Autodesk Inventor part; units mm, degrees
ref_plane "YZ Plane" through (0, 0, 0) normal (1, 0, 0) x (0, 1, 0)
ref_plane "XZ Plane" through (0, 0, 0) normal (0, 1, 0) x (-1, 0, 0)
ref_plane "XY Plane" through (0, 0, 0) normal (0, 0, 1) x (1, 0, 0)
sketch "Sketch1" plane through (0, 0, 0) normal (0, 0, 1) x (1, 0, 0)
  line L0 (0, 273.8452) -> (193.6378, 193.6378) construction
  line L1 (193.6378, 193.6378) -> (273.8452, 0) construction
  line L2 (273.8452, 0) -> (193.6378, -193.6378) construction
  line L3 (193.6378, -193.6378) -> (0, -273.8452) construction
  line L4 (0, -273.8452) -> (-193.6378, -193.6378) construction
  line L5 (-193.6378, -193.6378) -> (-273.8452, 0) construction
  line L6 (-273.8452, 0) -> (-193.6378, 193.6378) construction
  line L7 (-193.6378, 193.6378) -> (0, 273.8452)
  line L8 (-193.6378, 193.6378) -> (0, 273.8452)
  line L9 (-459.9272, 770.6562) -> (-219.7185, 870.1539)
  line L10 (-96.8189, 233.7415) -> (-339.8229, 820.405) construction
  line L11 (-219.7185, 870.1539) -> (0, 870.1539)
  line L12 (0, 870.1539) -> (0, 273.8452)
  line L13 (-459.9272, 770.6562) -> (-615.2917, 615.2917)
  line L14 (-615.2917, 615.2917) -> (-193.6378, 193.6378)
  point P0 (0, 0)
  point P1 (0, 0)
  dimension "d0" = 506
  dimension "d2" = 260
  dimension "d3" = 635
extrude "Extrusion1" add sketch "Sketch1" along normal mid plane 0.5
sketch "Sketch7" plane through (0, 0, 0.25) normal (0, 0, 1) x (1, 0, 0)
  line L0 (-13, 865.1539) -> (-5, 865.1539)
  line L1 (-5, 865.1539) -> (-5, 857.1539)
  line L2 (-5, 857.1539) -> (-13, 857.1539)
  line L3 (-13, 857.1539) -> (-13, 865.1539)
  line L4 (0, 870.1539) -> (-219.7185, 870.1539)
  line L5 (0, 273.8452) -> (0, 870.1539)
  point P0 (0, 0)
  dimension "d54" = 8
  dimension "d55" = 8
  dimension "d56" = 5
  dimension "d57" = 5
extrude "Extrusion5" [suppressed]
pattern_linear "Rectangular Pattern1" [suppressed]
equation "\"d0\" = Барабан_габарит_по_кассетам"
equation "\"d2\" = Кассета_длина_грани"
equation "\"d3\" = Кассета_высота"
equation "\"BendRadius\" = Thickness"
equation "\"BendReliefWidth\" = Thickness"
equation "\"BendReliefDepth\" = 0.5 * Thickness"
equation "\"CornerReliefSize\" = 4 * Thickness"
equation "\"MinimumRemnant\" = 2 * Thickness"
equation "\"TransitionRadius\" = BendRadius"
equation "\"JacobiRadiusSize\" = BendRadius"
equation "\"GapSize\" = Thickness"
properties part number "ДМС 207 Сетка кассеты"
Check sheet for the modelled part. Datum: model origin and axes. Units: mm. Give positions to 0.01 mm unless a question says otherwise; leave off trailing zeros. Write each loop counter-clockwise with the first axis right and the second up, starting at its lowest first coordinate (ties: lowest second). Pieces come first, ordered by that corner, then holes.
Item 1: Cross-section at A-A (z = 0.1). Enter the section's corners in (x, y).
Item 2: Cross-section at C-C (y = 292.5). Enter the section's corners in (x, z), and give its area (3 significant figures).
Item 3: Gauge pin test, flat end, axial feed: pin 1 (12 mm diameter, centred on x = -507.5, y = 735.5, fed in from +Z). Record the tip position at first contact, or that the pin passes through.
Item 4: Scan lines: L1, parallel to Y at x = -306.5, z = -0.05; L2, parallel to X at y = 448, z = -0.15; L3, parallel to X at y = 785, z = -0.2. Record each from-to range of solid material in increasing order.
Item 5: Cross-section at B-B (x = -205). Enter the section's corners in (y, z).
Report:
1. outline: (-615.29, 615.29) - (-193.64, 193.64) - (0, 273.85) - (0, 870.15) - (-219.72, 870.15) - (-459.93, 770.66) - close
2. outline: (-292.5, -0.25) - (0, -0.25) - (0, 0.25) - (-292.5, 0.25) - close
2. area: 146 mm2
3. pin 1: passes through
4. L1: y = 306.5 to 834.21
4. L2: x = -448 to 0
4. L3: x = -425.3 to 0
5. outline: (205, -0.25) - (870.15, -0.25) - (870.15, 0.25) - (205, 0.25) - close
